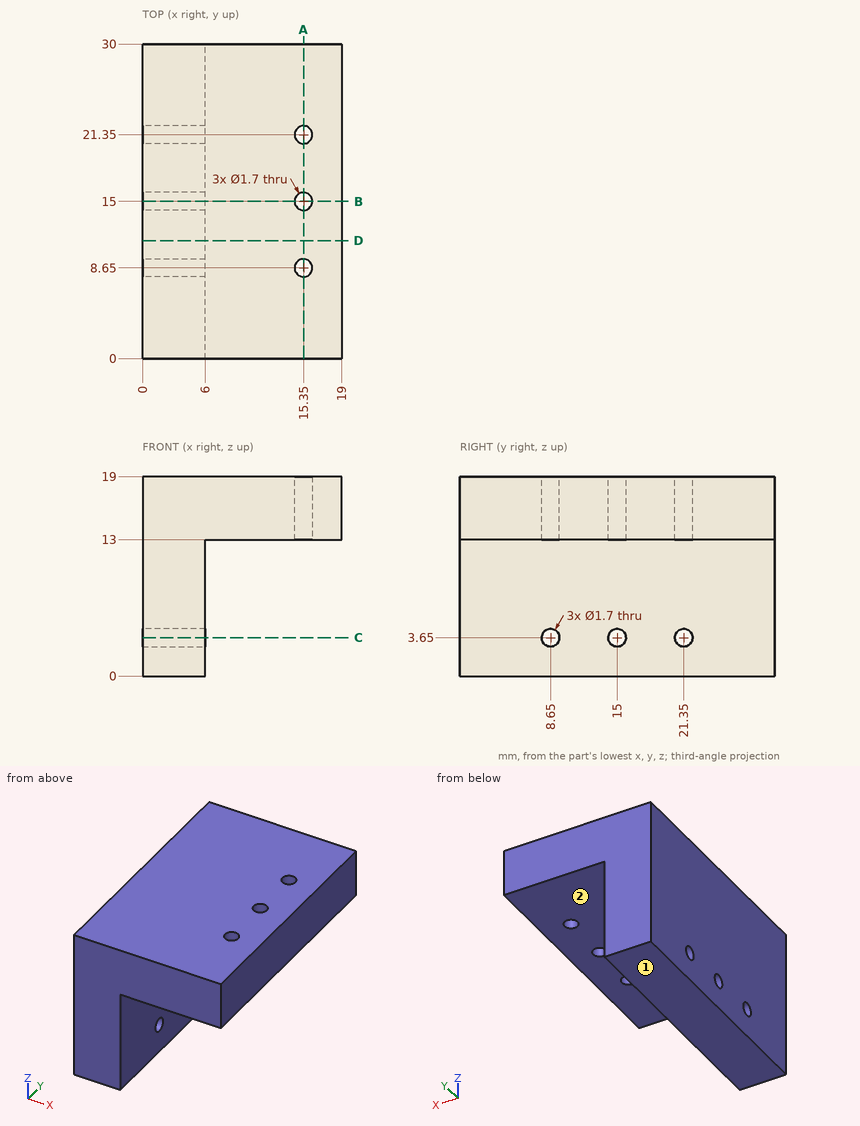
Input: dimensioned drawing with shaded views. Units: mm. Origin: part minimum x, y, z. A direction names the side the tool comes from. Round coordinates to 2 decimals unless told otherwise and drop trailing zeros. Order: outer loops, then holes, each group sorted by start corner. A loop starts at its lowest first (then second) coordinate and runs counter-clockwise, first axis right, second up. Notation, with made-up numbers: (35, 54) - (43, 54) arc R15 cw to (43, 76) - close; hole circle Ø1 at (11.5, 13.25). An arc over 180 degrees is marked (long way). Write item = value, one per line. Start each with the question number.
Q1. Cut plane C-C on z = 3.65. Return the cut outline in (x, y), and give its area (3 significant figures).
Q2. Cut plane B-B on y = 15. Return the cut outline in (x, z).
Q3. Cut plane D-D on y = 11.25. Return the cut outline in (x, z).
Q4. Cut plane A-A on x = 15.35. Return the cut outline in (y, z), and give its area (3 significant figures).
Q5. Ray query, line 1 (Y direction, x = 2.25, z = 3.65); line 2 (Z direction, x = 1.5, y = 21.35); line 3 (Z direction, x = 10, y = 8.75). Return the intervals inside material, ascending. Write a range as from..to.
Q6. Pin query (flat end, axial travel): pin 1 (1 mm diameter, centred on x = 14, z = 11, fed in from +Y); pin 2 (6.5 mm diameter, centred on x = 9.5, y = 14, fed in from -Z); pin 3 (2 mm diameter, centred on y = 15, z = 3.65, fed in from +X). Return the tip coordinate at first contact, or that it passes through.
Q7. Access query for the marked faces 1 and 2. Directions: +Z, -Z, +X, -X, +Y, -Y. A direction counts if a zero-diameter tool reaches every point of the face in a straight line with its end or side. Return the directions, or none.
Outcome:
q1.outline = (0, 0) - (6, 0) - (6, 7.8) - (0, 7.8) - close; (0, 9.5) - (6, 9.5) - (6, 14.15) - (0, 14.15) - close; (0, 15.85) - (6, 15.85) - (6, 20.5) - (0, 20.5) - close; (0, 22.2) - (6, 22.2) - (6, 30) - (0, 30) - close
q1.area = 149 mm^2
q2.outline = (0, 0) - (6, 0) - (6, 2.8) - (0, 2.8) - close; (0, 4.5) - (6, 4.5) - (6, 13) - (14.5, 13) - (14.5, 19) - (0, 19) - close; (16.2, 13) - (19, 13) - (19, 19) - (16.2, 19) - close
q3.outline = (0, 0) - (6, 0) - (6, 13) - (19, 13) - (19, 19) - (0, 19) - close
q4.outline = (0, 13) - (7.8, 13) - (7.8, 19) - (0, 19) - close; (9.5, 13) - (14.15, 13) - (14.15, 19) - (9.5, 19) - close; (15.85, 13) - (20.5, 13) - (20.5, 19) - (15.85, 19) - close; (22.2, 13) - (30, 13) - (30, 19) - (22.2, 19) - close
q4.area = 149 mm^2
q5.line_1 = 0..7.8, 9.5..14.15, 15.85..20.5, 22.2..30
q5.line_2 = 0..2.8, 4.5..19
q5.line_3 = 13..19
q6.pin_1 = through
q6.pin_2 = 13
q6.pin_3 = 6
q7.face_1 = -Z, +X, -X, +Y, -Y
q7.face_2 = -Z, +X, +Y, -Y
